```python
from build123d import *

# Parameters (mm, degrees)
SKETCH_1_R          = 17.5
SKETCH_1_R_2        = 1.5
EXTRUDE_1_DEPTH     = 2
EXTRUDE_2_DEPTH     = 6
SKETCH_5_R          = 3
CUT_EXTRUDE_1_DEPTH = 1


with BuildPart() as part:
    # 草图1 → 凸台-拉伸1 (new body)
    with BuildSketch(Plane(origin=(0, 0, 0), x_dir=(1, 0, 0), z_dir=(0, 1, 0))):
        with Locations(Location((0, 0, 0), (0, 0, 270))):
            Circle(SKETCH_1_R)
        with Locations(Location((0, -13.5, 0), (0, 0, 270))):
            Circle(SKETCH_1_R_2, mode=Mode.SUBTRACT)
        with Locations(Location((-11.691342951, -6.75, 0), (0, 0, 270))):
            Circle(SKETCH_1_R_2, mode=Mode.SUBTRACT)
        with Locations(Location((-11.691342951, 6.75, 0), (0, 0, 270))):
            Circle(SKETCH_1_R_2, mode=Mode.SUBTRACT)
        with Locations(Location((0, 13.5, 0), (0, 0, 270))):
            Circle(SKETCH_1_R_2, mode=Mode.SUBTRACT)
        with Locations(Location((11.691342951, 6.75, 0), (0, 0, 270))):
            Circle(SKETCH_1_R_2, mode=Mode.SUBTRACT)
        with Locations(Location((11.691342951, -6.75, 0), (0, 0, 270))):
            Circle(SKETCH_1_R_2, mode=Mode.SUBTRACT)
    extrude(amount=EXTRUDE_1_DEPTH)

    # 草图4 → 凸台-拉伸2 (add)
    with BuildSketch(Plane.XZ):
        Polygon((-2.985497273, 3.681012496), (-4.738451875, 0.10060218), (-3.681012496, -2.985497273), (-0.10060218, -4.738451875), (2.985497273, -3.681012496), (4.738451875, -0.10060218), (3.681012496, 2.985497273), (0.10060218, 4.738451875), align=None)
        with BuildLine():
            Line((-0.412394562, 2.97706408), (-1.500063983, 2.604378593))
            ThreePointArc((-1.500063983, 2.604378593), (-1.854278529, 2.39852018), (-2.102751494, 2.072779767))
            Line((-2.102751494, 2.072779767), (-2.926796788, 0.389666998))
            ThreePointArc((-2.926796788, 0.389666998), (-3.031700416, -0.006364389), (-2.97706408, -0.412394562))
            Line((-2.97706408, -0.412394562), (-2.604378593, -1.500063983))
            ThreePointArc((-2.604378593, -1.500063983), (-2.39852018, -1.854278529), (-2.072779767, -2.102751494))
            Line((-2.072779767, -2.102751494), (-0.389666998, -2.926796788))
            ThreePointArc((-0.389666998, -2.926796788), (0.006364389, -3.031700416), (0.412394562, -2.97706408))
            Line((0.412394562, -2.97706408), (1.500063983, -2.604378593))
            ThreePointArc((1.500063983, -2.604378593), (1.854278529, -2.39852018), (2.102751494, -2.072779767))
            Line((2.102751494, -2.072779767), (2.926796788, -0.389666998))
            ThreePointArc((2.926796788, -0.389666998), (3.031700416, 0.006364389), (2.97706408, 0.412394562))
            Line((2.97706408, 0.412394562), (2.604378593, 1.500063983))
            ThreePointArc((2.604378593, 1.500063983), (2.39852018, 1.854278529), (2.072779767, 2.102751494))
            Line((2.072779767, 2.102751494), (0.389666998, 2.926796788))
            ThreePointArc((0.389666998, 2.926796788), (-0.006364389, 3.031700416), (-0.412394562, 2.97706408))
        make_face(mode=Mode.SUBTRACT)
    extrude(amount=EXTRUDE_2_DEPTH)

    # 草图5 → 切除-拉伸1 (cut)
    with BuildSketch(Plane.XZ):
        with Locations(Location((-11.691342951, 6.75, 0), (0, 0, 270))):
            Circle(SKETCH_5_R)
        with Locations(Location((0, 13.5, 0), (0, 0, 270))):
            Circle(SKETCH_5_R)
        with Locations(Location((11.691342951, 6.75, 0), (0, 0, 270))):
            Circle(SKETCH_5_R)
        with Locations(Location((11.691342951, -6.75, 0), (0, 0, 270))):
            Circle(SKETCH_5_R)
        with Locations(Location((0, -13.5, 0), (0, 0, 270))):
            Circle(SKETCH_5_R)
        with Locations(Location((-11.691342951, -6.75, 0), (0, 0, 270))):
            Circle(SKETCH_5_R)
    extrude(amount=-CUT_EXTRUDE_1_DEPTH, mode=Mode.SUBTRACT)


solid = part.part
```
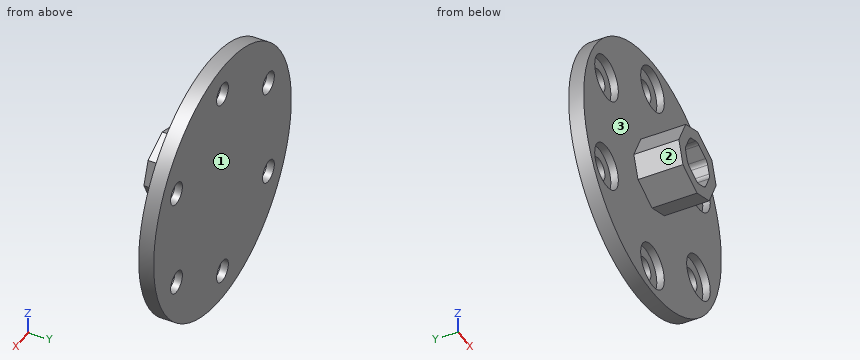
Can you work these out from the model? Positions are in its coordinate system, mm. Face numbers are marked on the shaded views. Coordinates: 2 decimals unless noted, no trailing zeros. Loops run counter-clockwise (first coordinate to the right, second up) from the corner with the lowest first, then second, coordinate; pieces in that order, holes last. Notation, with made-up numbers: (81.5, 89.25) - (120.5, 89.25) arc R25 ccw to (120.5, 110.25) - close; hole circle Ø2 at (48, 63.25). An arc over 180 degrees is marked (long way). Answer as CSV lines item,"result". Start each with the question number.
1) For pin 1 (1.5 mm diameter, centred on x = 12, y = 0, fed in from -Z); pin 2 (3.5 mm diameter, centred on x = 0, z = 13.5, fed in from -Y); pin 3 (1 mm diameter, centred on y = 1, z = -10, fed in from +X), each with a flat end and sliding along its axis, tell me the tip position at first contact or that it passes through.
2) Suppose I cut it at C-C (z = 13.5). Please give me the cut outline in (x, y), plus the area to 3 significant figures.
3) Suppose I cut it at A-A (y = -2.5). Please give me the cut outline in (x, z).
4) Thinking about a two-plate mould opening in Y: for the marked faces 1, 2 and 3, which applies, pulls with the +Y half, pulls with the -Y half, needs draft (parallel to the pull), parting line crosses it, or undercut?
5) Suppose I cut it at D-D (y = 0.5). Please give me the cut outline in (x, z).
6) I need wall thicknesses on line 1 (X direction, y = 1.35, z = -6.75); line 2 (X direction, y = 1.75, z = -5.5); line 3 (Y direction, x = 16.5, z = -5). Which ranges of each line are inside material? Lowest first, please. Write a range as from..to.
7) Suppose I cut it at B-B (z = -6.75). Please give me the cut outline in (x, y), plus the area to 3 significant figures.
Check result:
1,pin 1,"stops at z = -13.4"
1,pin 2,"stops at y = 1"
1,pin 3,"stops at x = 14.7"
2,outline,"(-11.14, 0) - (-3, 0) - (-3, 1) - (-1.5, 1) - (-1.5, 2) - (-11.14, 2) - close; (1.5, 1) - (3, 1) - (3, 0) - (11.14, 0) - (11.14, 2) - (1.5, 2) - close"
2,area,"35.5 mm²"
3,outline,"(-4.74, 0.1) - (-3.68, -2.99) - (-0.1, -4.74) - (2.99, -3.68) - (4.74, -0.1) - (3.68, 2.99) - (0.1, 4.74) - (-2.99, 3.68) - close; hole (-2.98, -0.41) - (-2.6, -1.5) arc R1.05 ccw to (-2.07, -2.1) - (-0.39, -2.93) arc R1.05 ccw to (0.41, -2.98) - (1.5, -2.6) arc R1.05 ccw to (2.1, -2.07) - (2.93, -0.39) arc R1.05 ccw to (2.98, 0.41) - (2.6, 1.5) arc R1.05 ccw to (2.07, 2.1) - (0.39, 2.93) arc R1.05 ccw to (-0.41, 2.98) - (-1.5, 2.6) arc R1.05 ccw to (-2.1, 2.07) - (-2.93, 0.39) arc R1.05 ccw to start"
4,face 1,"pulls with the +Y half"
4,face 2,"needs draft"
4,face 3,"pulls with the -Y half"
5,outline,"circle Ø35 at (0, 0); hole circle Ø6 at (-11.69, -6.75); hole circle Ø6 at (-11.69, 6.75); hole circle Ø6 at (0, -13.5); hole circle Ø6 at (0, 13.5); hole circle Ø6 at (11.69, -6.75); hole circle Ø6 at (11.69, 6.75)"
6,line 1,"x = -16.15..-13.19, -10.19..10.19, 13.19..16.15"
6,line 2,"x = -16.61..-12.52, -10.86..10.86, 12.52..16.61"
6,line 3,"y = 0..2"
7,outline,"(-16.15, 0) - (-14.69, 0) - (-14.69, 1) - (-13.19, 1) - (-13.19, 2) - (-16.15, 2) - close; (-10.19, 1) - (-8.69, 1) - (-8.69, 0) - (8.69, 0) - (8.69, 1) - (10.19, 1) - (10.19, 2) - (-10.19, 2) - close; (13.19, 1) - (14.69, 1) - (14.69, 0) - (16.15, 0) - (16.15, 2) - (13.19, 2) - close"
7,area,"46.6 mm²"
